Autodesk Inventor part; units mm, degrees
ref_plane "Start plane" through (0, 0, 0) normal (0, 0, 1) x (1, 0, 0)
ref_plane "End plane" through (0, 0, 800) normal (0, 0, 1) x (1, 0, 0)
ref_plane "Work Plane4" through (0, -1090, 0) normal (0, 0, -1) x (-1, 0, 0)
ref_plane "Start plane" through (0, 0, 0) normal (0, 0, 1) x (1, 0, 0)
ref_plane "End plane" through (0, 0, 800) normal (0, 0, 1) x (1, 0, 0)
sketch "Sketch" plane through (0, 0, 0) normal (0, 0, 1) x (1, 0, 0)
  line L0 (-10, -6) -> (-10, 6)
  line L1 (-6, 10) -> (6, 10)
  line L2 (10, 6) -> (10, -6)
  line L3 (6, -10) -> (-6, -10)
  arc A0 (-10, -6) -> (-6, -10) centre (-6, -6) ccw
  arc A1 (10, 6) -> (6, 10) centre (6, 6) ccw
  arc A2 (-6, 10) -> (-10, 6) centre (-6, 6) ccw
  arc A3 (6, -10) -> (10, -6) centre (6, -6) ccw
  arc A4 (-6, 8) -> (-8, 6) centre (-6, 6) ccw
  line L4 (-6, 8) -> (6, 8)
  arc A5 (8, 6) -> (6, 8) centre (6, 6) ccw
  line L5 (8, 6) -> (8, -6)
  arc A6 (6, -8) -> (8, -6) centre (6, -6) ccw
  line L6 (6, -8) -> (-6, -8)
  arc A7 (-8, -6) -> (-6, -8) centre (-6, -6) ccw
  line L7 (-8, -6) -> (-8, 6)
  line L8 (0, 15.1598) -> (0, -15.1598) construction
  line L9 (-15.1598, 0) -> (15.1598, 0) construction
  dimension "d7" = 4
  dimension "d9" = 20
  dimension "d11" = 20
  dimension "d12" = 2
  dimension "d15" = 10
  dimension "d16" = 10
extrude "Body" add sketch "Sketch" along normal up to surface (800 mm away) from surface at 0
sketch "Sketch3" plane through (0, 0, 0) normal (0, 0, 1) x (1, 0, 0)
  line L0 (0, 0) -> (10, 0)
ref_plane "Work Plane3" through (0, 0, 0) normal (0, -1, 0) x (1, 0, 0)
sketch "Sketch4" plane through (0, 0, 0) normal (0, -1, 0) x (1, 0, 0)
  line L0 (-2, 0) -> (12, 0)
  line L1 (-2, 800) -> (12, 800)
  dimension "d18" = 800
ref_plane "Work Plane4" through (0, -1090, 0) normal (0, 0, -1) x (-1, 0, 0)
split "Split1" plane through (0, -1090, 0) removes the side toward (0, 0, -1)
ref_plane "Work Plane5" through (10, 0, 0) normal (-0.7071, 0, -0.7071) x (-0.7071, 0, 0.7071)
split "Split2" plane through (10, 0, 0) removes the side toward (-0.7071, 0, -0.7071)
ref_plane "Work Plane6" through (10, 0, 800) normal (-0.7071, 0, 0.7071) x (0.7071, 0, 0.7071)
split "Split3" plane through (10, 0, 800) removes the side toward (-0.7071, 0, 0.7071)
ref_plane "Work Plane7" through (0, 10, 800) normal (0, 0, 1) x (1, 0, 0)
split "Split4" plane through (0, 10, 800) removes the side toward (0, 0, 1)
equation "\"d7\" = G_IR"
equation "\"d9\" = G_W"
equation "\"d11\" = G_H"
equation "\"d12\" = G_T"
equation "\"d15\" = 0.5 * d9"
equation "\"d16\" = 0.5 * d11"
equation "\"d3\" = G_L"
equation "\"G_W\" = 20"
equation "\"G_H\" = 20"
equation "\"G_T\" = 2"
equation "\"G_IR\" = 4"
equation "\"G_L\" = d18"
equation "\"G_OFFSET_START\" = 0"
equation "\"G_OFFSET_END\" = 0"
properties part number "ISO 4019 - 20x20x2 - 800" material "Steel, Mild"
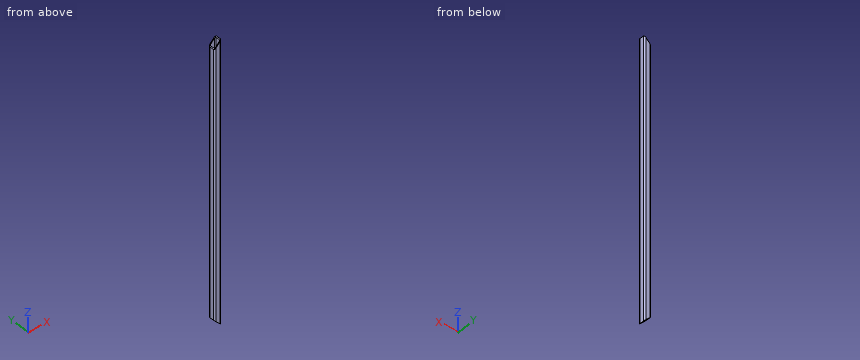
Build history of the part. All positions in model axes, mm. Round coordinates to 2 decimals unless told otherwise and drop trailing zeros. Loops run counter-clockwise (first coordinate to the right, second up) from the corner with the lowest first, then second, coordinate; pieces in that order, holes last. Notation, with made-up numbers: (-4, 7) -> (21, 7) arc R18 cw to (21, 37) -> close; hole circle Ø11 at (0.5, -39.5). An arc over 180 degrees is marked (long way). Use CSV: the item, a comma, the result in double quotes. Start each with the question number.
Q1. Flat gauge pins, fed straight in: pin 1 Ø8 at (x, y) = (-3.5, -4.5) entering from -Z; pin 2 Ø5 at (x, y) = (-0.5, 5) entering from +Z. Where does each tip first touch, or does it go through?
Q2. Saw through at C-C on y = 0.5. Give the cut face in (x, z).
Q3. Saw through at B-B on x = -2. Give the cut face in (y, z).
Q4. Drill centre lines: L1, parallel to Y at x = -4.25, z = 629; L2, parallel to X at y = 6.75, z = 351.5. Where is each one in solid material? Low to high.
Q5. Saw through at A-A on z = 403. Give the cut face in (x, y), and give its area (3 significant figures).
Solutions:
1,pin 1,"stops at z = 11.56"
1,pin 2,"passes through"
2,outline,"(-10, 20) -> (-8, 18) -> (-8, 782) -> (-10, 780) -> close; (8, 2) -> (10, 0) -> (10, 800) -> (8, 798) -> close"
3,outline,"(-10, 12) -> (-8, 12) -> (-8, 788) -> (-10, 788) -> close; (8, 12) -> (10, 12) -> (10, 788) -> (8, 788) -> close"
4,L1,"y = -10 to -8, 8 to 10"
4,L2,"x = -9.93 to -7.85, 7.85 to 9.93"
5,outline,"(-10, -6) arc R4 ccw to (-6, -10) -> (6, -10) arc R4 ccw to (10, -6) -> (10, 6) arc R4 ccw to (6, 10) -> (-6, 10) arc R4 ccw to (-10, 6) -> close; hole (-8, -6) arc R2 ccw to (-6, -8) -> (6, -8) arc R2 ccw to (8, -6) -> (8, 6) arc R2 ccw to (6, 8) -> (-6, 8) arc R2 ccw to (-8, 6) -> close"
5,area,"134 mm^2"
